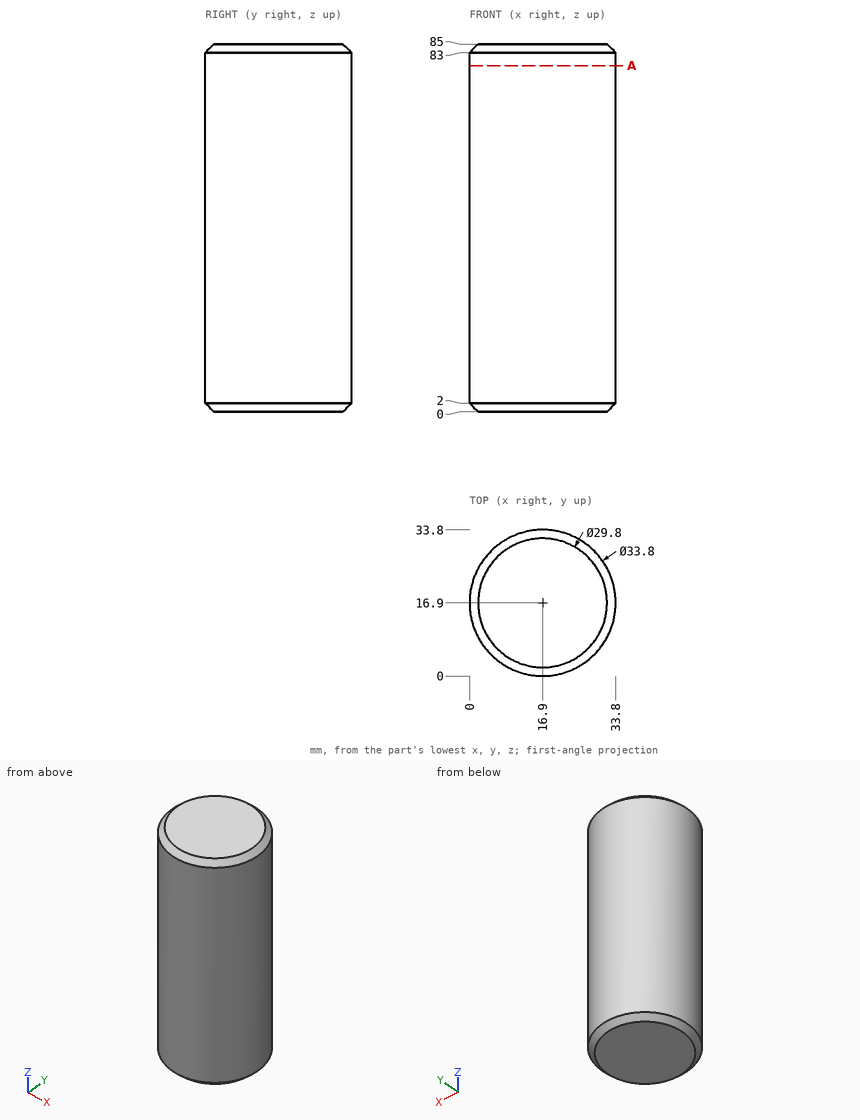
Check sheet for the drawn part. Datum: minimum x, y, z corner. Units: mm. Give positions to 0.01 mm unless a question says otherwise; leave off trailing zeros. Order: outer loops, then holes, each group sorted by start corner. A loop starts at its lowest first (then second) coordinate and runs counter-clockwise, first axis right, second up. Notation, with made-up numbers: (11, 34.5) - (58, 34.5) arc R23 cw to (58, 64.5) - close; hole circle Ø8 at (58.5, 12.5). An arc over 180 degrees is marked (long way). Write item = value, one per line. Start each with the question number.
1) Section check A-A (z = 80). Enter the section's corners in (x, y).
2) Scan lines: L1, parallel to Y at x = 17.5, z = 60; L2, parallel to Y at x = 28.5, z = 66.5. Record each from-to range of solid material in increasing order.
3) Gauge pin test, flat ends, axial feed: pin 1 Ø3 at (x, z) = (25.5, 64.5) entering from +Y; pin 2 Ø10 at (y, z) = (4, 31.5) entering from -X; pin 3 Ø1.5 at (x, z) = (26.5, 43) entering from -Y. Record the tip position at first contact, or that the pin passes through.
Geometry check:
q1.outline = circle Ø33.8 at (16.9, 16.9)
q2.L1 = 0.01 to 33.79
q2.L2 = 4.61 to 29.19
q3.pin_1 = 32.24
q3.pin_2 = 1.96
q3.pin_3 = 2.5
